Autodesk Fusion 360 part; units mm, degrees
sketch "Sketch1" plane through (0, 0, 0) normal (0, 0, 1) x (1, 0, 0)
  line L0 (40.8554, 59.6943) -> (40.8554, -37.5959)
  line L1 (-41.8946, 59.6943) -> (40.8554, 59.6943)
  line L2 (-41.8946, -37.5959) -> (-41.8946, 59.6943)
  line L3 (40.8554, -37.5959) -> (-41.8946, -37.5959)
  line L4 (-25.4246, 28.1391) -> (-12.4246, 28.1391)
  line L5 (-25.4246, 14.1391) -> (-12.4246, 14.1391)
  line L6 (-25.9246, 27.6391) -> (-25.9246, 14.6391)
  line L7 (-11.9246, 27.6391) -> (-11.9246, 14.6391)
  arc A0 (-25.4246, 28.1391) -> (-25.9246, 27.6391) centre (-25.4246, 27.6391) ccw
  arc A1 (-11.9246, 27.6391) -> (-12.4246, 28.1391) centre (-12.4246, 27.6391) ccw
  arc A2 (-25.9246, 14.6391) -> (-25.4246, 14.1391) centre (-25.4246, 14.6391) ccw
  arc A3 (-12.4246, 14.1391) -> (-11.9246, 14.6391) centre (-12.4246, 14.6391) ccw
  line L8 (-6.3746, 28.1391) -> (6.6254, 28.1391)
  line L9 (-6.3746, 14.1391) -> (6.6254, 14.1391)
  line L10 (-6.8746, 27.6391) -> (-6.8746, 14.6391)
  line L11 (7.1254, 27.6391) -> (7.1254, 14.6391)
  arc A4 (-6.3746, 28.1391) -> (-6.8746, 27.6391) centre (-6.3746, 27.6391) ccw
  arc A5 (7.1254, 27.6391) -> (6.6254, 28.1391) centre (6.6254, 27.6391) ccw
  arc A6 (-6.8746, 14.6391) -> (-6.3746, 14.1391) centre (-6.3746, 14.6391) ccw
  arc A7 (6.6254, 14.1391) -> (7.1254, 14.6391) centre (6.6254, 14.6391) ccw
  line L12 (12.6754, 28.1391) -> (25.6754, 28.1391)
  line L13 (12.6754, 14.1391) -> (25.6754, 14.1391)
  line L14 (12.1754, 27.6391) -> (12.1754, 14.6391)
  line L15 (26.1754, 27.6391) -> (26.1754, 14.6391)
  arc A8 (12.6754, 28.1391) -> (12.1754, 27.6391) centre (12.6754, 27.6391) ccw
  arc A9 (26.1754, 27.6391) -> (25.6754, 28.1391) centre (25.6754, 27.6391) ccw
  arc A10 (12.1754, 14.6391) -> (12.6754, 14.1391) centre (12.6754, 14.6391) ccw
  arc A11 (25.6754, 14.1391) -> (26.1754, 14.6391) centre (25.6754, 14.6391) ccw
  line L16 (-25.4246, 9.0891) -> (-12.4246, 9.0891)
  line L17 (-25.4246, -4.9109) -> (-12.4246, -4.9109)
  line L18 (-25.9246, 8.5891) -> (-25.9246, -4.4109)
  line L19 (-11.9246, 8.5891) -> (-11.9246, -4.4109)
  arc A12 (-25.4246, 9.0891) -> (-25.9246, 8.5891) centre (-25.4246, 8.5891) ccw
  arc A13 (-11.9246, 8.5891) -> (-12.4246, 9.0891) centre (-12.4246, 8.5891) ccw
  arc A14 (-25.9246, -4.4109) -> (-25.4246, -4.9109) centre (-25.4246, -4.4109) ccw
  arc A15 (-12.4246, -4.9109) -> (-11.9246, -4.4109) centre (-12.4246, -4.4109) ccw
  line L20 (-6.3746, 9.0891) -> (6.6254, 9.0891)
  line L21 (-6.3746, -4.9109) -> (6.6254, -4.9109)
  line L22 (-6.8746, 8.5891) -> (-6.8746, -4.4109)
  line L23 (7.1254, 8.5891) -> (7.1254, -4.4109)
  arc A16 (-6.3746, 9.0891) -> (-6.8746, 8.5891) centre (-6.3746, 8.5891) ccw
  arc A17 (7.1254, 8.5891) -> (6.6254, 9.0891) centre (6.6254, 8.5891) ccw
  arc A18 (-6.8746, -4.4109) -> (-6.3746, -4.9109) centre (-6.3746, -4.4109) ccw
  arc A19 (6.6254, -4.9109) -> (7.1254, -4.4109) centre (6.6254, -4.4109) ccw
  line L24 (12.6754, 9.0891) -> (25.6754, 9.0891)
  line L25 (12.6754, -4.9109) -> (25.6754, -4.9109)
  line L26 (12.1754, 8.5891) -> (12.1754, -4.4109)
  line L27 (26.1754, 8.5891) -> (26.1754, -4.4109)
  arc A20 (12.6754, 9.0891) -> (12.1754, 8.5891) centre (12.6754, 8.5891) ccw
  arc A21 (26.1754, 8.5891) -> (25.6754, 9.0891) centre (25.6754, 8.5891) ccw
  arc A22 (12.1754, -4.4109) -> (12.6754, -4.9109) centre (12.6754, -4.4109) ccw
  arc A23 (25.6754, -4.9109) -> (26.1754, -4.4109) centre (25.6754, -4.4109) ccw
  line L28 (-25.4246, -9.9609) -> (-12.4246, -9.9609)
  line L29 (-25.4246, -23.9609) -> (-12.4246, -23.9609)
  line L30 (-25.9246, -10.4609) -> (-25.9246, -23.4609)
  line L31 (-11.9246, -10.4609) -> (-11.9246, -23.4609)
  arc A24 (-25.4246, -9.9609) -> (-25.9246, -10.4609) centre (-25.4246, -10.4609) ccw
  arc A25 (-11.9246, -10.4609) -> (-12.4246, -9.9609) centre (-12.4246, -10.4609) ccw
  arc A26 (-25.9246, -23.4609) -> (-25.4246, -23.9609) centre (-25.4246, -23.4609) ccw
  arc A27 (-12.4246, -23.9609) -> (-11.9246, -23.4609) centre (-12.4246, -23.4609) ccw
  line L32 (-6.3746, -9.9609) -> (6.6254, -9.9609)
  line L33 (-6.3746, -23.9609) -> (6.6254, -23.9609)
  line L34 (-6.8746, -10.4609) -> (-6.8746, -23.4609)
  line L35 (7.1254, -10.4609) -> (7.1254, -23.4609)
  arc A28 (-6.3746, -9.9609) -> (-6.8746, -10.4609) centre (-6.3746, -10.4609) ccw
  arc A29 (7.1254, -10.4609) -> (6.6254, -9.9609) centre (6.6254, -10.4609) ccw
  arc A30 (-6.8746, -23.4609) -> (-6.3746, -23.9609) centre (-6.3746, -23.4609) ccw
  arc A31 (6.6254, -23.9609) -> (7.1254, -23.4609) centre (6.6254, -23.4609) ccw
  line L36 (12.6754, -9.9609) -> (25.6754, -9.9609)
  line L37 (12.6754, -23.9609) -> (25.6754, -23.9609)
  line L38 (12.1754, -10.4609) -> (12.1754, -23.4609)
  line L39 (26.1754, -10.4609) -> (26.1754, -23.4609)
  arc A32 (12.6754, -9.9609) -> (12.1754, -10.4609) centre (12.6754, -10.4609) ccw
  arc A33 (26.1754, -10.4609) -> (25.6754, -9.9609) centre (25.6754, -10.4609) ccw
  arc A34 (12.1754, -23.4609) -> (12.6754, -23.9609) centre (12.6754, -23.4609) ccw
  arc A35 (25.6754, -23.9609) -> (26.1754, -23.4609) centre (25.6754, -23.4609) ccw
  line L40 (9.2304, 48.2841) -> (21.7304, 48.2841)
  line L41 (21.7304, 48.2841) -> (21.7304, 35.7841)
  line L42 (21.7304, 35.7841) -> (9.2304, 35.7841)
  line L43 (9.2304, 35.7841) -> (9.2304, 48.2841)
  line L44 (-20.5696, 59.6943) -> (-2.0696, 59.6943)
  line L45 (-2.0696, 59.6943) -> (-2.0696, 38.1943)
  line L46 (-2.0696, 38.1943) -> (-20.5696, 38.1943)
  line L47 (-20.5696, 38.1943) -> (-20.5696, 59.6943)
  circle A36 centre (-36.8946, 54.6943) radius 1.45
  circle A37 centre (35.8554, 54.6943) radius 1.45
  circle A38 centre (35.8554, -32.5959) radius 1.45
  circle A39 centre (-36.8946, -32.5959) radius 1.45
  dimension "d1" = 14.68
  dimension "d2" = 13.635
  dimension "d3" = 12.5
  dimension "d4" = 12.5
  dimension "d5" = 19.125
  dimension "d6" = 7.645
  dimension "d7" = 18.5
  dimension "d8" = 21.5
  dimension "d9" = 11.3
  dimension "d10" = 2.9
  dimension "d11" = 5
  dimension "d12" = 5
  dimension "d13" = 2.9
  dimension "d14" = 5
  dimension "d15" = 5
  dimension "d16" = 2.9
  dimension "d17" = 5
  dimension "d18" = 5
  dimension "d19" = 2.9
  dimension "d20" = 5
  dimension "d21" = 5
extrude "Extrude1" add sketch "Sketch1" along normal blind 7 contours L0 L1 L2 L3 L45 L46 L47
fillet "Fillet1" radius 5 4 edges at (-41.8946, 59.6943, 3.5) (-41.8946, -37.5959, 3.5) (40.8554, -37.5959, 3.5) (40.8554, 59.6943, 3.5)
For this review, take the finished solid that the model builds, in its own axes (mm). A direction names the side the tool comes from. Round coordinates to 2 decimals unless told otherwise and drop trailing zeros. Write each loop counter-clockwise with the first axis right and the second up, starting at its lowest first coordinate (ties: lowest second). Pieces come first, ordered by that corner, then holes. Notation, with made-up numbers: (-37, 23) - (-10, 23) arc R15 cw to (-10, 35) - close; hole circle Ø10 at (-15, 19.5). An arc over 180 degrees is marked (long way). Put each result on its own line as item: value.
Q1. We need section A-A (x = -13.5). Give the boundary of the cut face in (y, z), and give its area (3 significant figures).
Solved:
outline: (-37.6, 0) - (-23.96, 0) - (-23.96, 7) - (-37.6, 7) - close; (-9.96, 0) - (-4.91, 0) - (-4.91, 7) - (-9.96, 7) - close; (9.09, 0) - (14.14, 0) - (14.14, 7) - (9.09, 7) - close; (28.14, 0) - (38.19, 0) - (38.19, 7) - (28.14, 7) - close
area: 237 mm2
Q2. Insertion check: pin 1 Ø3.5 at (x, z) = (-18.5, 5) entering from +Y. The pin has a flat end and moves straight along its axis. Give the tip position at first contact, or say it passes through.
Solved:
pin 1: stops at y = 38.19
Q3. Wall thickness on probe 1 along X at (y, z) = (1.5, 5.25); probe 2 along Y at (x, z) = (-14, 4.5); probe 3 along Y at (x, z) = (6, 4.5): over which ranges is each line inside the solid? List them lowest first.
Solved:
probe 1: x = -41.89 to -25.92, -11.92 to -6.87, 7.13 to 12.18, 26.18 to 40.86
probe 2: y = -37.6 to -23.96, -9.96 to -4.91, 9.09 to 14.14, 28.14 to 38.19
probe 3: y = -37.6 to -23.96, -9.96 to -4.91, 9.09 to 14.14, 28.14 to 59.69
Q4. We need section C-C (z = 5.25). Count the separate pieces of the cut face and the enclosed holes in it, and give its area (3 significant figures).
Solved:
separate pieces: 1
enclosed holes: 14
area: 5,690 mm2
Q5. Mouldability with a two-part tool opening along Y and no side actions: class faces 3 (the face through (-41.895, 10, 3)), 4 (the face through (12.175, -17, 3)), 5 (the face through (39.43, 58.19, 3.55)) as released by +Y, released by -Y, zero draft, split by the parting line, or undercut.
Solved:
face 3: zero draft
face 4: undercut
face 5: released by +Y
Q6. Machinability: for faces 1 (the face through (19, 14.139, 3)), 2 (the face through (40.855, 12, 3)), which of the approach directions +Z, -Z, +X, -X, +Y, -Y give a long, thin tool a straight path to every point of the face, cutting with its end or side? Answer none if there is none.
Solved:
face 1: +Z, -Z
face 2: +Z, -Z, +X, +Y, -Y
Q7. We need section B-B (y = -12.5). Give the boundary of the cut face in (x, z).
Solved:
outline: (-41.89, 0) - (-25.92, 0) - (-25.92, 7) - (-41.89, 7) - close; (-11.92, 0) - (-6.87, 0) - (-6.87, 7) - (-11.92, 7) - close; (7.13, 0) - (12.18, 0) - (12.18, 7) - (7.13, 7) - close; (26.18, 0) - (40.86, 0) - (40.86, 7) - (26.18, 7) - close
